```python
from build123d import *

# Parameters (mm, degrees)
BASE_FLANGE1_DEPTH   = 119.6975
EDGE_FLANGE1_DEPTH   = 119.6975
EDGE_FLANGE2_DEPTH   = 119.6975
EDGE_FLANGE2_2_DEPTH = 119.6975


# Read off the part's stored shape, not the designer's step: Edge-Flange2
# Sheet-metal steps are written as plain solids
with BuildPart() as part:
    # Sketch1 → Base-Flange1 (new body)
    with BuildSketch(Plane.XY):
        with BuildLine():
            ThreePointArc((-50.8, 170.388379885), (-142.557146436, 106.25582337), (-177.8, 0))
            Line((-177.8, 0), (-180.45684, 0))
            ThreePointArc((-180.45684, 0), (-144.68735751, 107.843588959), (-51.559097143, 172.934469105))
            Line((-51.559097143, 172.934469105), (-50.8, 170.388379885))
        make_face()
    extrude(amount=BASE_FLANGE1_DEPTH)

    # Edge-Flange1 section (across the edge) → Edge-Flange1 (add)
    with BuildSketch(Plane(origin=(-49.291175996, 173.610632552, 119.6975), x_dir=(-0.9999999996342678, -2.7045604981568168e-05, 0), z_dir=(0, 0, -1))):
        with BuildLine():
            Line((-2.65684, 2.366572064), (-2.65684, 74.219652496))
            Line((-2.65684, 74.219652496), (0, 74.219652496))
            Line((0, 74.219652496), (0, 2.366572064))
            ThreePointArc((0, 2.366572064), (0.62936233, 0.469112223), (2.267939433, -0.676102109))
            Line((2.267939433, -0.676102109), (1.508911151, -3.222211858))
            ThreePointArc((1.508911151, -3.222211858), (-1.500827273, -1.118682173), (-2.65684, 2.366572064))
        make_face()
    extrude(amount=EDGE_FLANGE1_DEPTH)

    # Edge-Flange2 outline → Edge-Flange2 (cut)
    with BuildSketch(Plane.XY):
        with BuildLine():
            Line((-46.636343312, 247.830356877), (-47.036345835, 247.830346059))
            ThreePointArc((-47.036345835, 247.830346059), (-46.737188142, 246.787726569), (-46.636285905, 245.707740707))
            Line((-46.636285905, 245.707740707), (-46.636343312, 247.830356877))
        make_face()
    extrude(amount=EDGE_FLANGE2_DEPTH, mode=Mode.SUBTRACT)

    # Edge-Flange2 2 outline → Edge-Flange2 2 (add)
    with BuildSketch(Plane.XY):
        with BuildLine():
            ThreePointArc((-47.036345835, 247.830346059), (-47.452236843, 248.682682095), (-48.000778663, 249.456338298))
            Line((-48.000778663, 249.456338298), (-111.945669395, 325.658705996))
            Line((-111.945669395, 325.658705996), (-113.980880724, 323.950867119))
            Line((-113.980880724, 323.950867119), (-50.035989993, 247.748499421))
            ThreePointArc((-50.035989993, 247.748499421), (-49.484631202, 246.793577627), (-49.293125904, 245.707668851))
            Line((-49.293125904, 245.707668851), (-49.293183311, 247.830285021))
            Line((-49.293183311, 247.830285021), (-47.036345835, 247.830346059))
        make_face()
    extrude(amount=EDGE_FLANGE2_2_DEPTH)


solid = part.part
```
Work out the finished part from the listing and answer in its coordinate system (mm). A direction names the side the tool comes from. Round coordinates to 2 decimals unless told otherwise and drop trailing zeros. Write each loop counter-clockwise with the first axis right and the second up, starting at its lowest first coordinate (ties: lowest second). Pieces come first, ordered by that corner, then holes. Notation, with made-up numbers: (69, 70) -> (74, 70) arc R16 cw to (74, 93) -> close; hole circle Ø7 at (50.25, 69). An arc over 180 degrees is marked (long way). Write each question's results on one line, items separated by ' | '.
1) The part is cut by section B-B (x = -89). Write down the section's boundary in (y, z), and give its area (3 significant figures).
Findings:
outline: (153.92, 0) -> (156.98, 0) -> (156.98, 119.7) -> (153.92, 119.7) -> close; (294.18, 0) -> (298.31, 0) -> (298.31, 119.7) -> (294.18, 119.7) -> close | area: 861 mm²
2) Consider line 1 along Y through (x, z) = (-78, 65); line 2 along Y through (x, z) = (-92.5, 8); line 3 along X through (y, z) = (208.5, 41). Determine where each line is inside the solid, lowest interval first. Write a range as [from, to].
Findings:
line 1: y = [159.78, 162.73], [281.07, 285.21] | line 2: y = [151.84, 154.95], [298.35, 302.49] | line 3: x = [-49.29, -46.64]
3) Which of the six approach directions +Z, -Z, +X, -X, +Y, -Y give full straight-line access (tool end or side, diameter ignored) to faces 1 (the flat face through (-94, 152, 119.698)), 2 (the cylindrical face through (-145.65, 106.54, 59.01))?
Findings:
face 1: +Z, +X, -X, +Y, -Y | face 2: +Z, -Z, -X
4) Flat-ended cylindrical pins translate along their axes: pin 1 (6 mm diameter, centred on y = 137, z = 39, fed in from +X); pin 2 (8 mm diameter, centred on y = 61, z = 105, fed in from +X); pin 3 (3 mm diameter, centred on x = -116.5, z = 94.5, fed in from +Y). Find the tip coordinate at first contact, or state that the pin passes through.
Findings:
pin 1: stops at x = -109.6 | pin 2: stops at x = -165.49 | pin 3: stops at y = 139.07
5) The part is cut by section D-D (x = -148). Write down the section's boundary in (y, z), and give its area (3 significant figures).
Findings:
outline: (98.53, 0) -> (103.25, 0) -> (103.25, 119.7) -> (98.53, 119.7) -> close | area: 565 mm²
6) The part is cut by section C-C (y = 164). Write down the section's boundary in (x, z), and give its area (3 significant figures).
Findings:
outline: (-75.29, 0) -> (-68.68, 0) -> (-68.68, 119.7) -> (-75.29, 119.7) -> close | area: 791 mm²
